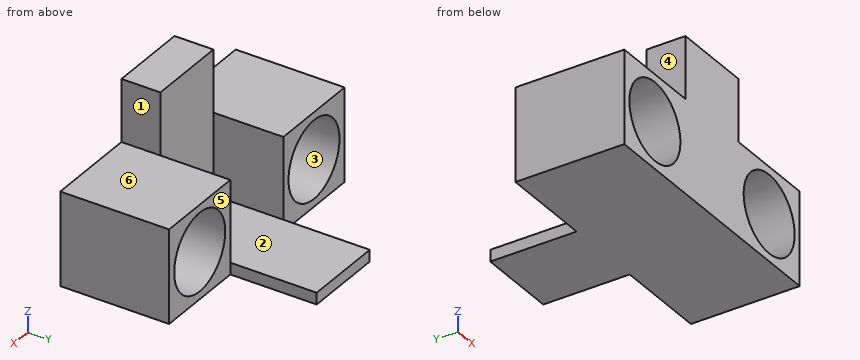
from build123d import *

# Parameters (mm, degrees)
F0_W     = 104
F0_H     = 200
F1_DEPTH = 50
F2_W     = 120
F2_H     = 120
F3_DEPTH = 140
F4_R     = 50
F5_DEPTH = 140.001
F7_DEPTH = 15


with BuildPart() as f1:
    # F0 (on Front) → F1 (new body)
    with BuildSketch(Plane.XZ):
        with Locations((-47.456343, 24.031783)):
            Rectangle(F0_W, F0_H)
    extrude(amount=F1_DEPTH)

    # F2 (on face) → F3 (join)
    with BuildSketch(Plane.XZ.offset(50)):
        with Locations((-159.456343, -15.968217)):
            Rectangle(F2_W, F2_H)
        with Locations((64.543657, -15.968217)):
            Rectangle(F2_W, F2_H)
    extrude(amount=-F3_DEPTH)

    # F4 (on face) → F5 (cut, through all)
    with BuildSketch(Plane(origin=(0, 90, 0), x_dir=(-1, 0, 0), z_dir=(0, 1, 0))):
        with Locations((-64.543657, -15.968217)):
            Circle(F4_R)
        with Locations((159.456343, -15.968217)):
            Circle(F4_R)
    extrude(amount=-F5_DEPTH, mode=Mode.SUBTRACT)

    # F6 (on face) → F7 (join)
    with BuildSketch(Plane(origin=(0, 0, -75.968217), x_dir=(1, 0, 0), z_dir=(0, 0, -1))):
        Polygon((0, 0), (-99.456343, 0), (-99.456343, -90), (-99.456343, -201.058388), (4.543657, -201.058388), (4.543657, -90), (4.543657, 0), align=None)
    extrude(amount=-F7_DEPTH)


solid = f1.part
Part model, mm, in its own coordinate system. Face numbers are marked on the shaded views. A direction names the side the tool comes from. Give positions to 0.01 mm unless a question says otherwise; leave off trailing zeros. Loops run counter-clockwise (first coordinate to the right, second up) from the corner with the lowest first, then second, coordinate; pieces in that order, holes last. Notation, with made-up numbers: M 66.25,43 L 71.25,43 A14 cw 71.25,57 Z; hole C 48.5,11 d8. An arc over 180 degrees is marked long. Put each result on its own line as item: value. Start each with the question number.
1) Saw through at B-B (z = 3.5). List the corners of the cut face in (x, y).
2) Saw through at A-A (x = -115.5). List the corners of the cut face in (y, z).
3) Probe probe 1 along X at (y, z) = (21, -48); probe 2 along Z at (x, y) = (67.5, 25.5); probe 3 along X at (y, z) = (-5.5, 83). List the from-to ranges inside material, lowest first.
4) Saw through at D-D (x = 50.5). List the corners of the cut face in (y, z), then the cut area to 3 significant figures.
5) Flat gauge pins, fed straight in: pin 1 (1.5 mm diameter, centred on x = -94.5, y = 153.5, fed in from +Z); pin 2 (16.5 mm diameter, centred on y = 131.5, z = -67, fed in from +X); pin 3 (6 mm diameter, centred on x = -56.5, z = -23.5, fed in from +Y). Where does each tip first touch, or does it go through?
6) Saw through at C-C (y = 4.5). List the corners of the cut face in (x, z).
7) Pull direction Z, two halves, no side cores. Call the marked faces 1, 2 and 3: +Z half, -Z half, draft (parallel to the pull), parting line (faces both ways), or undercut.
8) 3-axis set-ups, long thin cutter, end or side, ignore diameter. For the marked faces 4, 5 and 6: which of +Z, -Z, +X, -X, +Y, -Y reach the whole face in a straight line?
Numbers:
1. outline: M -219.46,-50 L -205.51,-50 L -205.51,90 L -219.46,90 Z; M -113.4,-50 L 18.49,-50 L 18.49,90 L 4.54,90 L 4.54,0 L -99.46,0 L -99.46,90 L -113.4,90 Z; M 110.6,-50 L 124.54,-50 L 124.54,90 L 110.6,90 Z
2. outline: M -50,-75.97 L 90,-75.97 L 90,-39.8 L -50,-39.8 Z; M -50,7.86 L 90,7.86 L 90,44.03 L -50,44.03 Z
3. probe 1: -219.46 to -197.85, -121.06 to -99.46, 4.54 to 26.15, 102.94 to 124.54
3. probe 2: -75.97 to -65.88, 33.94 to 44.03
3. probe 3: -99.46 to 4.54
4. outline: M -50,-75.97 L 90,-75.97 L 90,-63.96 L -50,-63.96 Z; M -50,32.02 L 90,32.02 L 90,44.03 L -50,44.03 Z
4. area: 3,360 mm^2
5. pin 1: z = -60.97
5. pin 2: x = 4.54
5. pin 3: y = 0
6. outline: M -219.46,-75.97 L 124.54,-75.97 L 124.54,44.03 L 4.54,44.03 L 4.54,-60.97 L -99.46,-60.97 L -99.46,44.03 L -219.46,44.03 Z; hole C -159.46,-15.97 d100; hole C 64.54,-15.97 d100
7. face 1: draft
7. face 2: +Z half
7. face 3: undercut
8. face 4: +Z, -X, +Y, -Y
8. face 5: +Z, -Z, +X, +Y
8. face 6: +Z, +X, +Y, -Y
